```python
from build123d import *

# Parameters (mm, degrees)
F0_R     = 101.6
F0_R_2   = 3.175
F1_DEPTH = 6.35


# Not quite as in the source:
# - the program builds the solid bodies; features that only make, move or delete a surface that nothing else refers to are left out


with BuildPart() as f1:
    # F0 (on Top) → F1 (new body)
    with BuildSketch(Plane.XY):
        with Locations((1.0160004022, -0.2540000132)):
            Circle(F0_R)
        with Locations((-62.8617928475, -62.8617928475)):
            Circle(F0_R_2, mode=Mode.SUBTRACT)
        with Locations((-34.0205571373, -82.1328904403)):
            Circle(F0_R_2, mode=Mode.SUBTRACT)
        with Locations((0, -88.9)):
            Circle(F0_R_2, mode=Mode.SUBTRACT)
        with Locations((-24.3003979552, -58.6663503145)):
            Circle(F0_R_2, mode=Mode.SUBTRACT)
        with Locations((0, -63.5)):
            Circle(F0_R_2, mode=Mode.SUBTRACT)
        with Locations((-82.1328904403, -34.0205571373)):
            Circle(F0_R_2, mode=Mode.SUBTRACT)
        with Locations((-58.6663503145, -24.3003979552)):
            Circle(F0_R_2, mode=Mode.SUBTRACT)
        with Locations((-44.9012806053, -44.9012806053)):
            Circle(F0_R_2, mode=Mode.SUBTRACT)
        with Locations((-26.9407683632, -26.9407683632)):
            Circle(F0_R_2, mode=Mode.SUBTRACT)
        with Locations((-14.5802387731, -35.1998101887)):
            Circle(F0_R_2, mode=Mode.SUBTRACT)
        with Locations((0, -38.1)):
            Circle(F0_R_2, mode=Mode.SUBTRACT)
        with Locations((-35.1998101887, -14.5802387731)):
            Circle(F0_R_2, mode=Mode.SUBTRACT)
        with Locations((0, -12.7)):
            Circle(F0_R_2, mode=Mode.SUBTRACT)
        with Locations((34.0205571373, -82.1328904403)):
            Circle(F0_R_2, mode=Mode.SUBTRACT)
        with Locations((24.3003979552, -58.6663503145)):
            Circle(F0_R_2, mode=Mode.SUBTRACT)
        with Locations((62.8617928475, -62.8617928475)):
            Circle(F0_R_2, mode=Mode.SUBTRACT)
        with Locations((14.5802387731, -35.1998101887)):
            Circle(F0_R_2, mode=Mode.SUBTRACT)
        with Locations((44.9012806053, -44.9012806053)):
            Circle(F0_R_2, mode=Mode.SUBTRACT)
        with Locations((26.9407683632, -26.9407683632)):
            Circle(F0_R_2, mode=Mode.SUBTRACT)
        with Locations((35.1998101887, -14.5802387731)):
            Circle(F0_R_2, mode=Mode.SUBTRACT)
        with Locations((82.1328904403, -34.0205571373)):
            Circle(F0_R_2, mode=Mode.SUBTRACT)
        with Locations((58.6663503145, -24.3003979552)):
            Circle(F0_R_2, mode=Mode.SUBTRACT)
        with Locations((-88.9, 0)):
            Circle(F0_R_2, mode=Mode.SUBTRACT)
        with Locations((-63.5, 0)):
            Circle(F0_R_2, mode=Mode.SUBTRACT)
        with Locations((-58.6663503145, 24.3003979552)):
            Circle(F0_R_2, mode=Mode.SUBTRACT)
        with Locations((-82.1328904403, 34.0205571373)):
            Circle(F0_R_2, mode=Mode.SUBTRACT)
        with Locations((-38.1, 0)):
            Circle(F0_R_2, mode=Mode.SUBTRACT)
        with Locations((-35.1998101887, 14.5802387731)):
            Circle(F0_R_2, mode=Mode.SUBTRACT)
        with Locations((-12.7, 0)):
            Circle(F0_R_2, mode=Mode.SUBTRACT)
        Circle(F0_R_2, mode=Mode.SUBTRACT)
        with Locations((0, 12.7)):
            Circle(F0_R_2, mode=Mode.SUBTRACT)
        with Locations((-26.9407683632, 26.9407683632)):
            Circle(F0_R_2, mode=Mode.SUBTRACT)
        with Locations((-44.9012806053, 44.9012806053)):
            Circle(F0_R_2, mode=Mode.SUBTRACT)
        with Locations((-14.5802387731, 35.1998101887)):
            Circle(F0_R_2, mode=Mode.SUBTRACT)
        with Locations((0, 38.1)):
            Circle(F0_R_2, mode=Mode.SUBTRACT)
        with Locations((-62.8617928475, 62.8617928475)):
            Circle(F0_R_2, mode=Mode.SUBTRACT)
        with Locations((-24.3003979552, 58.6663503145)):
            Circle(F0_R_2, mode=Mode.SUBTRACT)
        with Locations((0, 63.5)):
            Circle(F0_R_2, mode=Mode.SUBTRACT)
        with Locations((-34.0205571373, 82.1328904403)):
            Circle(F0_R_2, mode=Mode.SUBTRACT)
        with Locations((0, 88.9)):
            Circle(F0_R_2, mode=Mode.SUBTRACT)
        with Locations((12.7, 0)):
            Circle(F0_R_2, mode=Mode.SUBTRACT)
        with Locations((38.1, 0)):
            Circle(F0_R_2, mode=Mode.SUBTRACT)
        with Locations((35.1998101887, 14.5802387731)):
            Circle(F0_R_2, mode=Mode.SUBTRACT)
        with Locations((14.5802387731, 35.1998101887)):
            Circle(F0_R_2, mode=Mode.SUBTRACT)
        with Locations((26.9407683632, 26.9407683632)):
            Circle(F0_R_2, mode=Mode.SUBTRACT)
        with Locations((44.9012806053, 44.9012806053)):
            Circle(F0_R_2, mode=Mode.SUBTRACT)
        with Locations((63.5, 0)):
            Circle(F0_R_2, mode=Mode.SUBTRACT)
        with Locations((58.6663503145, 24.3003979552)):
            Circle(F0_R_2, mode=Mode.SUBTRACT)
        with Locations((88.9, 0)):
            Circle(F0_R_2, mode=Mode.SUBTRACT)
        with Locations((82.1328904403, 34.0205571373)):
            Circle(F0_R_2, mode=Mode.SUBTRACT)
        with Locations((24.3003979552, 58.6663503145)):
            Circle(F0_R_2, mode=Mode.SUBTRACT)
        with Locations((34.0205571373, 82.1328904403)):
            Circle(F0_R_2, mode=Mode.SUBTRACT)
        with Locations((62.8617928475, 62.8617928475)):
            Circle(F0_R_2, mode=Mode.SUBTRACT)
    extrude(amount=F1_DEPTH)


solid = f1.part
```
The listing builds one solid part. Answer for the finished solid, in the listing's coordinates (mm). Round coordinates to 2 decimals unless told otherwise and drop trailing zeros. Loops run counter-clockwise (first coordinate to the right, second up) from the corner with the lowest first, then second, coordinate; pieces in that order, holes last. Notation, with made-up numbers: (4, 41) - (61, 41) arc R11 ccw to (61, 46) - close; hole circle Ø3 at (45, -24.75). An arc over 180 degrees is marked (long way). Use one line per item in the form item = value. Start each with the question number.
1. Consider line 1 (Y direction, x = -63.5, z = 5.75) (3 decimals); line 2 (Y direction, x = 38, z = 5); line 3 (X direction, y = -42.5, z = 4.5). Determine where each line is inside the solid, lowest interval first. Write a range as [from, to].
2. Given pin 1 Ø1 at (x, z) = (-43.5, 3.5) entering from -Y; pin 2 Ø1.5 at (y, z) = (-73.5, 2.5) entering from -X, each flat-ended and moving along its own axis, determine where each tip first touches the part or whether it passes through.
3. The part is cut by section A-A on y = -88.9. Determine the outline of the cut face in (x, z) (3 decimals), then the cut area to 3 significant figures.
4. The part is cut by section C-C on z = 2.75. Give the number of separate pieces and of enclosed holes in the cut face, then the cut area to 3 significant figures.
5. The part is cut by section B-B on x = 82.5. Determine the outline of the cut face in (y, z), then the cut area to 3 significant figures.
6. For a pull along X with two mould halves and no side action, classify faces 1 (the face through (46.608, 47.578, 3.131)), 2 (the face through (22, 1, 0)) as pulls with the +X half, pulls with the -X half, needs draft (parallel to the pull), parting line crosses it, or undercut.
Geometry check:
q1.line_1 = [-78.741, -65.972], [-59.752, -3.175], [3.175, 59.752], [65.972, 78.233]
q1.line_2 = [-94.88, -16.08], [-13.08, -3.17], [3.17, 13.08], [16.08, 94.38]
q1.line_3 = [-91.38, -46.98], [-42.82, 42.82], [46.98, 93.42]
q2.pin_1 = -91.82
q2.pin_2 = -70.17
q3.outline = (-48.627, 0) - (-3.175, 0) - (-3.175, 6.35) - (-48.627, 6.35) - close; (3.175, 0) - (50.659, 0) - (50.659, 6.35) - (3.175, 6.35) - close
q3.area = 590 mm^2
q4.separate_pieces = 1
q4.enclosed_holes = 53
q4.area = 30,800 mm^2
q5.outline = (-60.94, 0) - (-37.17, 0) - (-37.17, 6.35) - (-60.94, 6.35) - close; (-30.87, 0) - (30.87, 0) - (30.87, 6.35) - (-30.87, 6.35) - close; (37.17, 0) - (60.43, 0) - (60.43, 6.35) - (37.17, 6.35) - close
q5.area = 691 mm^2
q6.face_1 = undercut
q6.face_2 = needs draft
